from build123d import *

# Parameters (mm, degrees)
SKETCH1_W           = 16
SKETCH1_H           = 16
BOSS_EXTRUDE1_DEPTH = 6.35
BOSS_EXTRUDE2_START = 6.35
SKETCH1_3_R         = 2.425
BOSS_EXTRUDE2_DEPTH = 2
SKETCH2_R           = 1.55
BOSS_EXTRUDE3_DEPTH = 6


with BuildPart() as part:
    # Sketch1 → Boss-Extrude1 (new body)
    with BuildSketch(Plane(origin=(0, 0, 0), x_dir=(1, 0, 0), z_dir=(0, 1, 0))):
        Rectangle(SKETCH1_W, SKETCH1_H)
    extrude(amount=BOSS_EXTRUDE1_DEPTH)

    # Sketch1<3> → Boss-Extrude2 (add)
    with BuildSketch(Plane(origin=(0, 0, 0), x_dir=(1, 0, 0), z_dir=(0, 1, 0)).offset(BOSS_EXTRUDE2_START)):
        with Locations(Location((-3.975, -3.975, 0), (0, 0, 90))):
            Circle(SKETCH1_3_R)
        with Locations(Location((3.975, -3.975, 0), (0, 0, 90))):
            Circle(SKETCH1_3_R)
        with Locations(Location((3.975, 3.975, 0), (0, 0, 90))):
            Circle(SKETCH1_3_R)
        with Locations(Location((-3.975, 3.975, 0), (0, 0, 90))):
            Circle(SKETCH1_3_R)
    extrude(amount=BOSS_EXTRUDE2_DEPTH)

    # Sketch2 → Boss-Extrude3 (add)
    with BuildSketch(Plane(origin=(8, 0, 0), x_dir=(0, 0, -1), z_dir=(1, 0, 0))):
        with Locations((0, 4.3)):
            Circle(SKETCH2_R)
    extrude(amount=BOSS_EXTRUDE3_DEPTH)


solid = part.part
Geometry check sheet. Reference: the model listing, model coordinates, mm. A direction names the side the tool comes from. Round coordinates to 2 decimals unless told otherwise and drop trailing zeros. Order: outer loops, then holes, each group sorted by start corner. A loop starts at its lowest first (then second) coordinate and runs counter-clockwise, first axis right, second up. Notation, with made-up numbers: M 61,-25 L 119,-25 A22 cw 119,11 Z; hole C 2,48.5 d10. An arc over 180 degrees is marked long. Write each question's results on one line, items separated by ' | '. Start each with the question number.
1. Cross-section at B-B on y = 4.3. Record the boundary of the cut face in (x, z).
2. Cross-section at C-C on x = -5.75. Record the boundary of the cut face in (y, z), plus the area to 3 significant figures.
3. Set-up check for faces 1 (the face through (-2.5, 7.34, -2.05)), 2 (the face through (0, 3, -8)), 3 (the face through (10.958, 2.787, 0.336)): record each of +Z, -Z, +X, -X, +Y, -Y from which the full face is reachable in a straight line by a thin tool's end or side.
4. Material ranges on L1, parallel to X at y = 2, z = 1.5; L2, parallel to Y at x = -5, z = 1.5; L3, parallel to Z at x = 6, y = 6.5, recorded low to high. Write a range as from..to.
5. Cross-section at D-D on z = -3. Record the boundary of the cut face in (x, y).
6. Draft check along X on faces 4 (the face through (-1.608, 7.336, 4.501)), 5 (the face through (14, 4, 0)), 6 (the face through (-8, 3, 0)). Enter one of: pulls with the +X half, pulls with the -X half, needs draft (parallel to the pull), parting line crosses it, or undercut.
7. Cross-section at A-A on z = 0. Record the boundary of the cut face in (x, y), plus the area to 3 significant figures.
8. Go/stop test with a flat-tipped pin: P1, Ø4, axis at y = 3, z = -4, coming from the +X side. Record where the tip stops, or that it passes through.
Resolved:
1) outline: M -8,-8 L 8,-8 L 8,-1.55 L 14,-1.55 L 14,1.55 L 8,1.55 L 8,8 L -8,8 Z
2) outline: M 0,-8 L 6.35,-8 L 6.35,-5.63 L 8.35,-5.63 L 8.35,-2.32 L 6.35,-2.32 L 6.35,2.32 L 8.35,2.32 L 8.35,5.63 L 6.35,5.63 L 6.35,8 L 0,8 Z | area: 115 mm2
3) face 1: +Y | face 2: -Z, +X, -X, +Y, -Y | face 3: +X
4) L1: -8..8 | L2: 0..6.35 | L3: -5.31..-2.64, 2.64..5.31
5) outline: M -8,0 L 8,0 L 8,6.35 L 6.2,6.35 L 6.2,8.35 L 1.75,8.35 L 1.75,6.35 L -1.75,6.35 L -1.75,8.35 L -6.2,8.35 L -6.2,6.35 L -8,6.35 Z
6) face 4: undercut | face 5: pulls with the +X half | face 6: pulls with the -X half
7) outline: M -8,0 L 8,0 L 8,2.75 L 14,2.75 L 14,5.85 L 8,5.85 L 8,6.35 L -8,6.35 Z | area: 120 mm2
8) P1: x = 8
